Design review of the part built by this model. Coordinates are the model's own, in mm. Face numbers are marked on the shaded views. A direction names the side the tool comes from. Coordinates: 2 decimals unless noted, no trailing zeros. Write each loop counter-clockwise with the first axis right and the second up, starting at its lowest first coordinate (ties: lowest second). Pieces come first, ordered by that corner, then holes. Notation, with made-up numbers: M 68,-35.5 L 93,-35.5 A20 ccw 93,1.5 Z; hole C -11,23.25 d8. An arc over 180 degrees is marked long. Return JSON: item names as keys, results as strings. Group by question number.
```python
from build123d import *

# Parameters (mm, degrees)
EXTRUDE_THIN1_DEPTH   = 80
SKETCH5_R             = 4.1
SKETCH5_R_2           = 3
CUT_EXTRUDE2_DEPTH    = 10
SKETCH6_W             = 57.412547925
SKETCH6_H             = 40
CUT_EXTRUDE3_DEPTH    = 10
M8X1_0_TAPPED_HOLE3_D = 7


with BuildPart() as part:
    # Sketch1 → Extrude-Thin1 (new body)
    with BuildSketch(Plane(origin=(0, 0, 0), x_dir=(1, 0, 0), z_dir=(0, 1, 0))):
        with BuildLine():
            Line((-22.658959538, -16.878612717), (-22.658959538, 20.121387283))
            ThreePointArc((-22.658959538, 20.121387283), (-21.780279881, 22.242707627), (-19.658959538, 23.121387283))
            Line((-19.658959538, 23.121387283), (17.341040462, 23.121387283))
            Line((17.341040462, 23.121387283), (17.341040462, 19.121387283))
            Line((17.341040462, 19.121387283), (-18.658959538, 19.121387283))
            Line((-18.658959538, 19.121387283), (-18.658959538, -16.878612717))
            Line((-18.658959538, -16.878612717), (-22.658959538, -16.878612717))
        make_face()
    extrude(amount=EXTRUDE_THIN1_DEPTH)

    # Sketch5 → Cut-Extrude2 (cut)
    with BuildSketch(Plane.ZY.offset(22.658959538)):
        with Locations((-3.121387283, 20)):
            Circle(SKETCH5_R)
        with Locations((-3.121387283, 47.5)):
            Circle(SKETCH5_R_2)
        with Locations((-3.121387283, 72.5)):
            Circle(SKETCH5_R_2)
    extrude(amount=-CUT_EXTRUDE2_DEPTH, mode=Mode.SUBTRACT)

    # Sketch6 → Cut-Extrude3 (cut)
    with BuildSketch(Plane(origin=(0, 0, -23.121387283), x_dir=(-1, 0, 0), z_dir=(0, 0, -1))):
        with Locations((-10.047314424, 20)):
            Rectangle(SKETCH6_W, SKETCH6_H)
    extrude(amount=-CUT_EXTRUDE3_DEPTH, mode=Mode.SUBTRACT)

    # M8x1.0 Tapped Hole3 (through all)
    with Locations(Plane(origin=(0, 0, -23.121387283), x_dir=(-1, 0, 0), z_dir=(0, 0, -1))):
        with Locations((2.658959538, 67)):
            Hole(M8X1_0_TAPPED_HOLE3_D / 2)


solid = part.part
```
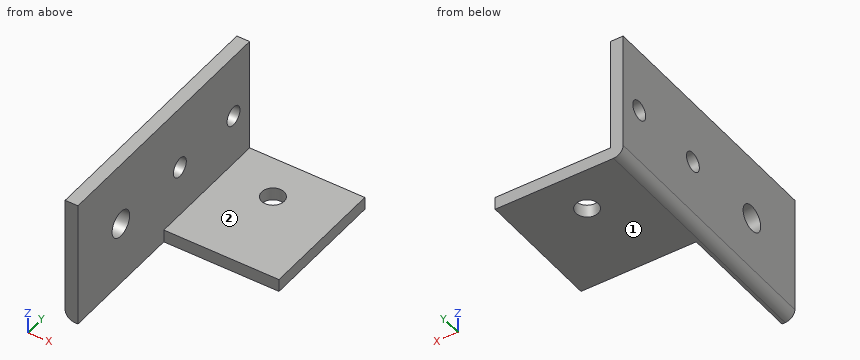
Item 1: Add section D-D (z = -13.5). Write out the cut boundary in (x, y), plus the area to 3 significant figures.
Item 2: For line 1 (X direction, y = 57, z = -13.5); line 2 (Z direction, x = 4, y = 75); line 3 (Y direction, x = -8.5, z = -19.5), list the stretches that pass through material, from the lowest coordinate up.
Item 3: For pin 1 (4 mm diameter, centred on y = 12.5, z = 4.5, fed in from +X); pin 2 (2 mm diameter, centred on x = 2.5, y = 47.5, fed in from +Z); pin 3 (2 mm diameter, centred on x = 6.5, z = -20.5, fed in from -Y), all flat-tipped, find the tip position at first contact; note any pin that passes through.
Item 4: Add section A-A (y = 67). Write out the cut boundary in (x, z), plus the area to 3 significant figures.
Item 5: Add section C-C (x = -9.5). Write out the cut boundary in (y, z).
Item 6: Add section B-B (y = 47.5). Write out the cut boundary in (x, z).
Item 7: Machinability: for the marked faces 1 and 2, which of the approach directions +Z, -Z, +X, -X, +Y, -Y give a long, thin tool a straight path to every point of the face, cutting with its end or side? Answer none if there is none.
Geometry check:
{
 "1": {"outline": "M -22.66,0 L -18.66,0 L -18.66,80 L -22.66,80 Z", "area": "320 mm^2"},
 "2": {"line 1": "-22.66 to -18.66", "line 2": "-23.12 to -19.12", "line 3": "40 to 80"},
 "3": {"pin 1": "x = -18.66", "pin 2": "z = -19.12", "pin 3": "y = 40"},
 "4": {"outline": "M -22.66,-20.12 A3 ccw -19.66,-23.12 L -6.16,-23.12 L -6.16,-19.12 L -18.66,-19.12 L -18.66,16.88 L -22.66,16.88 Z; M 0.84,-23.12 L 17.34,-23.12 L 17.34,-19.12 L 0.84,-19.12 Z", "area": "274 mm^2"},
 "5": {"outline": "M 40,-23.12 L 80,-23.12 L 80,-19.12 L 40,-19.12 Z"},
 "6": {"outline": "M -22.66,-20.12 A3 ccw -19.66,-23.12 L 17.34,-23.12 L 17.34,-19.12 L -18.66,-19.12 L -18.66,-6.12 L -22.66,-6.12 Z; M -22.66,-0.12 L -18.66,-0.12 L -18.66,16.88 L -22.66,16.88 Z"},
 "7": {"face 1": "-Z, +X, -X, +Y, -Y", "face 2": "+Z, +X, +Y, -Y"}
}
